Here's how the part is built. I have some questions about the finished solid (model axes, mm). A direction names the side the tool comes from. Coordinates: 2 decimals unless noted, no trailing zeros. Write each loop counter-clockwise with the first axis right and the second up, starting at its lowest first coordinate (ties: lowest second). Pieces come first, ordered by that corner, then holes. Notation, with made-up numbers: (-22.5, 1.25) -> (0.5, 1.25) arc R13 cw to (0.5, 14.25) -> close; hole circle Ø5 at (-31, -26). An arc over 180 degrees is marked (long way). Use a Markdown table: item, result. Add a question column.
Item 1: Will these pins go through, and if not, where does the flat tip stop? pin 1 Ø2 at (x, z) = (89, 0) entering from -Y (3 decimals); pin 2 Ø5 at (x, y) = (45.5, -4.5) entering from +Z; pin 3 Ø10 at (x, z) = (125, 19.5) entering from +Y; pin 4 Ø3 at (x, z) = (89, 4) entering from -Y.
Item 2: If we mould it in two halves opening along X, with no side actions, what happens to faces 3 (the cylindrical face through (166.246, 10.902, 3.433)), 4 (the conical face through (177.677, 8.597, 2.707)), 5 (the flat face through (157.48, -4, 9))? For each: pulls with the +X half, pulls with the -X half, needs draft (parallel to the pull), parting line crosses it, or undercut.
Item 3: Imagine slicing it at C-C, the plane x = 149. Write out the boundary of the cut face in (y, z) (3 decimals), and give its area (3 significant figures).
Item 4: Imagine slicing it at A-A, the plane y = 0. Write out the boundary of the cut face in (x, z) (3 decimals), and give its area (3 significant figures).
Item 5: If I drill on line 1 along X through (y, z) = (4, -20); line 2 along Y through (x, z) = (55, 4.5); line 3 along Z through (x, y) = (96, 1), over which ranges is the centre line in solid material (lowest first)? Write a range as from..to.
Item 6: On a 3-axis mill with a long thin cutter (end or side, diameter ignored), from which of +Z, -Z, +X, -X, +Y, -Y can I reach the whole of each face in a straight line? I mean faces 1 (the cylindrical face through (1.252, -5.506, -24.796)), 2 (the cylindrical face through (80.213, -7.559, -5.796)). Say none if no direction works.
```python
from build123d import *

# Parameters (mm, degrees)
F0_R     = 25.4
F1_DEPTH = 5.08
F2_R     = 2.54
F3_R     = 9.525
F4_DEPTH = 152.4
F5_R     = 11.43
F5_R_2   = 9.525
F6_DEPTH = 20.32
F7_SIZE  = 2.54


with BuildPart() as f1:
    # F0 (on Right) → F1 (new body)
    with BuildSketch(Plane.YZ):
        Circle(F0_R)
    extrude(amount=F1_DEPTH)

    # F2
    f2_edges = [f1.edges().sort_by_distance(p)[0] for p in [
        (5.08, -25.4, 0),
    ]]
    fillet(f2_edges, radius=F2_R)

    # F3 (on face) → F4 (join)
    with BuildSketch(Plane.YZ.offset(5.08)):
        Circle(F3_R)
    extrude(amount=F4_DEPTH)

    # F5 (on face) → F6 (join)
    with BuildSketch(Plane.YZ.offset(157.48)):
        Circle(F5_R)
        Circle(F5_R_2, mode=Mode.SUBTRACT)
        Circle(F5_R_2)
    extrude(amount=F6_DEPTH)

    # F7
    f7_edges = [f1.edges().sort_by_distance(p)[0] for p in [
        (177.8, -11.43, 0),
    ]]
    chamfer(f7_edges, length=F7_SIZE)


solid = f1.part
```
Ans:
| question | item | result |
|---|---|---|
| 1 | pin 1 | stops at y = -9.525 |
| 1 | pin 2 | stops at z = 9.31 |
| 1 | pin 3 | passes through |
| 1 | pin 4 | stops at y = -9.19 |
| 2 | face 3 | needs draft |
| 2 | face 4 | pulls with the +X half |
| 2 | face 5 | undercut |
| 3 | outline | circle Ø19.05 at (0, 0) |
| 3 | area | 285 mm^2 |
| 4 | outline | (0, -25.4) -> (2.54, -25.4) arc R2.54 ccw to (5.08, -22.86) -> (5.08, -9.525) -> (157.48, -9.525) -> (157.48, -11.43) -> (175.26, -11.43) -> (177.8, -8.89) -> (177.8, 8.89) -> (175.26, 11.43) -> (157.48, 11.43) -> (157.48, 9.525) -> (5.08, 9.525) -> (5.08, 22.86) arc R2.54 ccw to (2.54, 25.4) -> (0, 25.4) -> close |
| 4 | area | 3,620 mm^2 |
| 5 | line 1 | x = 0..5.08 |
| 5 | line 2 | y = -8.39..8.39 |
| 5 | line 3 | z = -9.47..9.47 |
| 6 | face 1 | +X, -X |
| 6 | face 2 | none |
